Can you work these out from the drawing? Everything is in mm from the part's minimum corner. A direction names the side the tool comes from. Coordinates: 2 decimals unless noted, no trailing zeros. Loops run counter-clockwise (first coordinate to the right, second up) from the corner with the lowest first, then second, coordinate; pieces in that order, holes last.
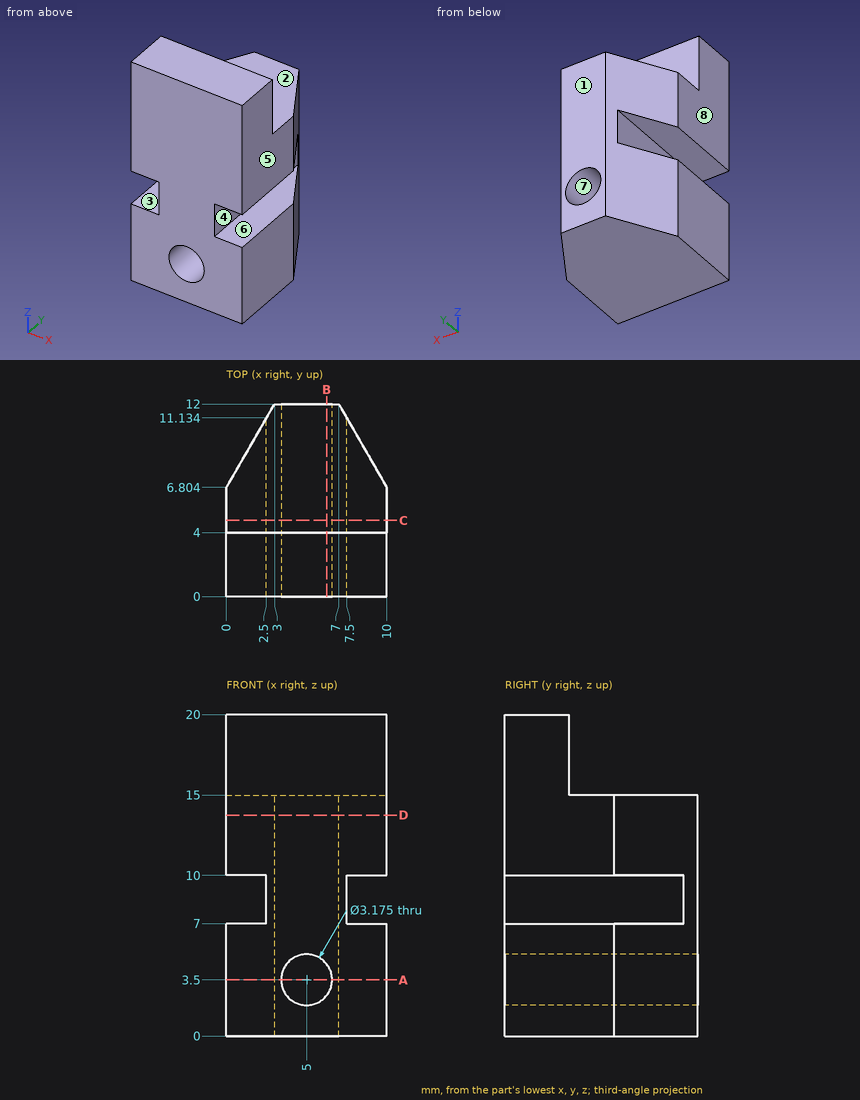
Item 1: Suppose I cut it at A-A, the plane z = 3.5. Please give me the cut outline in (x, y), plus the area to 3 significant figures.
Results are:
outline: (0, 0) - (3.41, 0) - (3.41, 12) - (3, 12) - (0, 6.8) - close; (6.59, 0) - (10, 0) - (10, 6.8) - (7, 12) - (6.59, 12) - close
area: 66.3 mm2
Item 2: We'd pull the mould along X, two halves only. Please class the marked faces 5, 6, 7 and 8: +X half, -X half, draft (parallel to the pull), parting line (faces both ways), or undercut.
Results are:
face 5: +X half
face 6: draft
face 7: undercut
face 8: -X half
Item 3: Suppose I cut it at D-D, the plane z = 13.75. Please give me the cut outline in (x, y).
Results are:
outline: (0, 0) - (10, 0) - (10, 6.8) - (7, 12) - (3, 12) - (0, 6.8) - close
Item 4: I need wall thicknesses on line 1 along Z through (x, y) = (5, 8.5); line 2 along Z through (x, y) = (1.75, 5.25); line 3 along Z through (x, y) = (6.75, 6.25). Which ranges of each line are inside material? Lowest first, please.
Results are:
line 1: z = 0 to 1.91, 5.09 to 15
line 2: z = 0 to 7, 10 to 15
line 3: z = 0 to 15
Item 5: Suppose I cut it at C-C, the plane y = 4.75. Please give me the cut outline in (x, z) (1 decimal), plus the area to 3 significant figures.
Results are:
outline: (0, 0) - (10, 0) - (10, 7) - (7.5, 7) - (7.5, 10) - (10, 10) - (10, 15) - (0, 15) - (0, 10) - (2.5, 10) - (2.5, 7) - (0, 7) - close; hole circle Ø3.2 at (5, 3.5)
area: 127 mm2
Item 6: On a 3-axis mill with a long thin cutter (end or side, diameter ignored), from which of +Z, -Z, +X, -X, +Y, -Y can I reach the whole of each face in a straight line? I mean the marked faces 1, 2, 3 and 4. Say none if no direction works.
Results are:
face 1: +Z, -Z, +X, -X, +Y
face 2: +Z, +X, -X, +Y
face 3: -X, +Y, -Y
face 4: +X, +Y, -Y
Item 7: I'm going to push flat-ended pins straight in: P1, Ø2, axis at x = 9, y = 6.5, coming from the +Z side; P2, Ø1, axis at x = 1.5, z = 5.5, coming from the +Y side; P3, Ø0.9, axis at y = 4, z = 8.5, coming from the +X side. Where does each tip first touch, or does it pass through?
Results are:
P1: stops at z = 15
P2: stops at y = 10.27
P3: stops at x = 7.5
Item 8: Suppose I cut it at B-B, the plane x = 6.25. Please give me the cut outline in (y, z), plus the area to 4 significant figures.
Results are:
outline: (0, 0) - (12, 0) - (12, 2.52) - (0, 2.52) - close; (0, 4.48) - (12, 4.48) - (12, 15) - (4, 15) - (4, 20) - (0, 20) - close
area: 176.5 mm2
